Source: CAD feature listing. Evaluate the final solid. Frame: model axes, mm. A direction names the side the tool comes from. Give positions to 0.01 mm unless a question says otherwise; leave off trailing zeros. Loops run counter-clockwise (first coordinate to the right, second up) from the corner with the lowest first, then second, coordinate; pieces in that order, holes last.
from build123d import *

# Parameters (mm, degrees)
F0_W          = 47
F0_H          = 29
F1_DEPTH      = 1.5
F0_R          = 1.65
F2_DEPTH      = 3
F3_W          = 41
F3_H          = 23
F4_DEPTH      = 1.5
F4_DEPTH_BACK = 25


with BuildPart() as f1:
    # F0 (on Top) → F1 (new body)
    with BuildSketch(Plane.XY):
        with Locations((0, 14.5)):
            Rectangle(F0_W, F0_H)
    extrude(amount=F1_DEPTH)

    # F0 (on Top) → F2 (join)
    with BuildSketch(Plane.XY):
        with BuildLine():
            ThreePointArc((-21.533361, 33.65), (-23.10973, 33.904996), (-24.525312, 34.643976))
            ThreePointArc((-24.525312, 34.643976), (-28.834444, 34.33246), (-29.142296, 30.023065))
            ThreePointArc((-29.142296, 30.023065), (-28.401441, 28.606095), (-28.145774, 27.027708))
            Line((-28.145774, 27.027708), (-28.145774, 1.972292))
            ThreePointArc((-28.145774, 1.972292), (-28.401441, 0.393905), (-29.142296, -1.023065))
            ThreePointArc((-29.142296, -1.023065), (-29.617954, -4.080909), (-27.351685, -6.188202))
            ThreePointArc((-27.351685, -6.188202), (-24.676504, -7.9735), (-23.642116, -11.018812))
            Line((-23.642116, -11.018812), (-23.642116, -12.65))
            ThreePointArc((-23.642116, -12.65), (-23.05633, -14.064214), (-21.642116, -14.65))
            Line((-21.642116, -14.65), (21.642116, -14.65))
            ThreePointArc((21.642116, -14.65), (23.05633, -14.064214), (23.642116, -12.65))
            Line((23.642116, -12.65), (23.642116, -11.018812))
            ThreePointArc((23.642116, -11.018812), (24.676504, -7.9735), (27.351685, -6.188202))
            ThreePointArc((27.351685, -6.188202), (29.617954, -4.080909), (29.142296, -1.023065))
            ThreePointArc((29.142296, -1.023065), (28.401441, 0.393905), (28.145774, 1.972292))
            Line((28.145774, 1.972292), (28.145774, 27.027708))
            ThreePointArc((28.145774, 27.027708), (28.401441, 28.606095), (29.142296, 30.023065))
            ThreePointArc((29.142296, 30.023065), (28.834444, 34.33246), (24.525312, 34.643976))
            ThreePointArc((24.525312, 34.643976), (23.10973, 33.904996), (21.533361, 33.65))
            Line((21.533361, 33.65), (-21.533361, 33.65))
        make_face()
        with Locations((-16.5, -11.65)):
            Circle(F0_R, mode=Mode.SUBTRACT)
        with Locations((-26.5, -3)):
            Circle(F0_R, mode=Mode.SUBTRACT)
        with Locations((16.5, -11.65)):
            Circle(F0_R, mode=Mode.SUBTRACT)
        with Locations((26.5, -3)):
            Circle(F0_R, mode=Mode.SUBTRACT)
        with BuildLine():
            ThreePointArc((-28.145774, 32.118016), (-26.440954, 33.648943), (-24.85, 32))
            ThreePointArc((-24.85, 32), (-26.440954, 30.351057), (-28.145774, 31.881984))
            ThreePointArc((-28.145774, 31.881984), (-28.15, 32), (-28.145774, 32.118016))
        make_face(mode=Mode.SUBTRACT)
        with Locations((0, 14.5)):
            Rectangle(F0_W, F0_H, mode=Mode.SUBTRACT)
        with BuildLine():
            ThreePointArc((28.145774, 32.118016), (28.148943, 32.059046), (28.15, 32))
            ThreePointArc((28.15, 32), (28.148943, 31.940954), (28.145774, 31.881984))
            ThreePointArc((28.145774, 31.881984), (24.85, 32), (28.145774, 32.118016))
        make_face(mode=Mode.SUBTRACT)
    extrude(amount=F2_DEPTH)

    # F3 (on face) → F4 (cut, two sides)
    with BuildSketch(Plane.XY.offset(1.5)) as f4_sk:
        with Locations((0, 14.5)):
            Rectangle(F3_W, F3_H)
    extrude(amount=-F4_DEPTH, mode=Mode.SUBTRACT)
    extrude(f4_sk.sketch, amount=-F4_DEPTH_BACK, mode=Mode.SUBTRACT)


solid = f1.part
1) Cut plane B-B (x = 11). Return loops of the section in (y, z), and give its area (3 significant figures).
Checks:
outline: (-14.65, 0) - (3, 0) - (3, 1.5) - (0, 1.5) - (0, 3) - (-14.65, 3) - close; (26, 0) - (33.65, 0) - (33.65, 3) - (29, 3) - (29, 1.5) - (26, 1.5) - close
area: 66.9 mm2
2) Cut plane C-C (y = 20). Return loops of the section in (x, z), and give its area (3 significant figures).
Checks:
outline: (-28.15, 0) - (-20.5, 0) - (-20.5, 1.5) - (-23.5, 1.5) - (-23.5, 3) - (-28.15, 3) - close; (20.5, 0) - (28.15, 0) - (28.15, 3) - (23.5, 3) - (23.5, 1.5) - (20.5, 1.5) - close
area: 36.9 mm2
3) Reachability of faces 1 (the flat face through (0, 3, 1)), 2 (the cylindrical face through (-23.1, 33.9, 1.5)), 3 (the cylindrical face through (28.4, 0.4, 1.5)), 4 (the flat face through (0, 2, 1.5)) from +Z, -Z, +X, -X, +Y, -Y: full face, straight path, thin tool, end or side. Return the list, or none.
Checks:
face 1: +Z, -Z
face 2: +Z, -Z, +Y
face 3: +Z, -Z, +X
face 4: +Z
4) Contact query for flat-ended pins moving along their axis: P1, Ø10, axis at x = 16, y = 21.5, coming from the +Z side; P2, Ø1.6, axis at y = 12.5, z = 1, coming from the -X side; P3, Ø1, axis at y = -5, z = 1.5, coming from the +X side; P4, Ø2.5, axis at x = 26.5, y = -3, coming from the +Z side. Output: stop coordinate, or through.
Checks:
P1: stops at z = 1.5
P2: stops at x = -28.15
P3: stops at x = 29.44
P4: passes through
5) Cut plane D-D (x = -16.5). Return loops of the section in (y, z).
Checks:
outline: (-14.65, 0) - (-13.3, 0) - (-13.3, 3) - (-14.65, 3) - close; (-10, 0) - (3, 0) - (3, 1.5) - (0, 1.5) - (0, 3) - (-10, 3) - close; (26, 0) - (33.65, 0) - (33.65, 3) - (29, 3) - (29, 1.5) - (26, 1.5) - close
6) Ray query, probe 1 along Y at (x, z) = (16.5, 1.15); probe 2 along Y at (x, z) = (16.5, 2.25); probe 3 along Y at (x, z) = (11, 2.65). Return the intervals inside material, ascending.
Checks:
probe 1: y = -14.65 to -13.3, -10 to 3, 26 to 33.65
probe 2: y = -14.65 to -13.3, -10 to 0, 29 to 33.65
probe 3: y = -14.65 to 0, 29 to 33.65
7) Pull-direction query (X, two-part tool) for faces 5 (the flat face through (-23.642, -12, 1)), 6 (the cylindrical face through (23.04, -14.08, 1.48)), 7 (the flat face through (0, 33.65, 1)), 8 (the flat face through (0, 0, 2)); classes: released by +X, released by -X, zero draft, split by the parting line, or undercut.
Checks:
face 5: released by -X
face 6: released by +X
face 7: undercut
face 8: undercut
8) Cut plane A-A (y = -3). Return loops of the section in (x, z).
Checks:
outline: (-29.8, 0) - (-28.15, 0) - (-28.15, 3) - (-29.8, 3) - close; (-24.85, 0) - (24.85, 0) - (24.85, 3) - (-24.85, 3) - close; (28.15, 0) - (29.8, 0) - (29.8, 3) - (28.15, 3) - close
